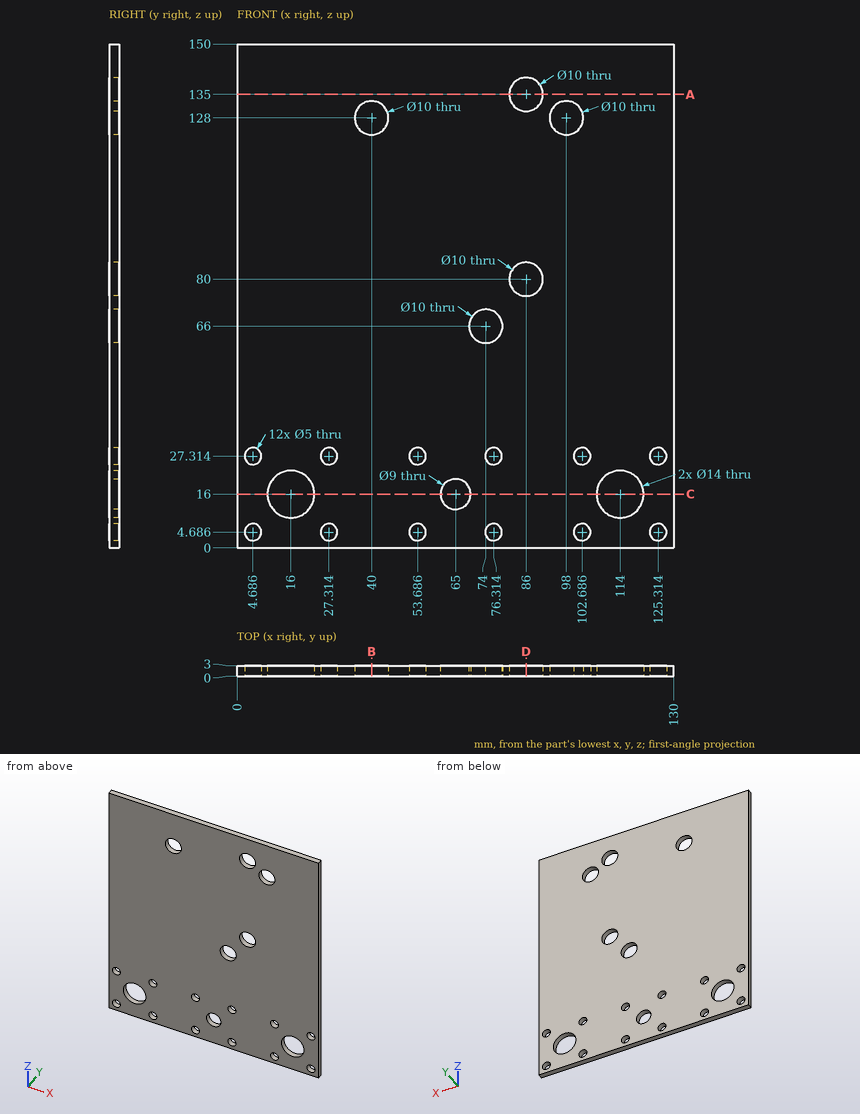
Geometry check sheet. Reference: drawing and pictorial views, mm from the part's lowest x, y, z. Round coordinates to 2 decimals unless told otherwise and drop trailing zeros. Loops run counter-clockwise (first coordinate to the right, second up) from the corner with the lowest first, then second, coordinate; pieces in that order, holes last. Notation, with made-up numbers: (83.25, -4.75) - (110.25, -4.75) arc R19 ccw to (110.25, 32.25) - close; hole circle Ø1 at (54.5, 41.5). An arc over 180 degrees is marked (long way). Answer in a Markdown table with one row per item. Add a question column.
Q1. Section check A-A on z = 135. Enter the section's corners in (x, y), plus the area to 3 significant figures.
Q2. Section check D-D on x = 86. Enter the section's corners in (y, z), plus the area to 3 significant figures.
Q3. Material ranges on line 1 (X direction, y = 0.95, z = 128); line 2 (Z direction, x = 65, y = 0.4); line 3 (X direction, y = 0.8, z = 80), recorded low to high.
Q4. Section check B-B on x = 40. Enter the section's corners in (y, z), plus the area to 3 significant figures.
Q5. Section check C-C on z = 16. Enter the section's corners in (x, y).
Found:
| question | item | result |
|---|---|---|
| 1 | outline | (0, 0) - (81, 0) - (81, 3) - (0, 3) - close; (91, 0) - (130, 0) - (130, 3) - (91, 3) - close |
| 1 | area | 360 mm² |
| 2 | outline | (0, 0) - (3, 0) - (3, 75) - (0, 75) - close; (0, 85) - (3, 85) - (3, 130) - (0, 130) - close; (0, 140) - (3, 140) - (3, 150) - (0, 150) - close |
| 2 | area | 390 mm² |
| 3 | line 1 | x = 0 to 35, 45 to 93, 103 to 130 |
| 3 | line 2 | z = 0 to 11.5, 20.5 to 150 |
| 3 | line 3 | x = 0 to 81, 91 to 130 |
| 4 | outline | (0, 0) - (3, 0) - (3, 123) - (0, 123) - close; (0, 133) - (3, 133) - (3, 150) - (0, 150) - close |
| 4 | area | 420 mm² |
| 5 | outline | (0, 0) - (9, 0) - (9, 3) - (0, 3) - close; (23, 0) - (60.5, 0) - (60.5, 3) - (23, 3) - close; (69.5, 0) - (107, 0) - (107, 3) - (69.5, 3) - close; (121, 0) - (130, 0) - (130, 3) - (121, 3) - close |
